from build123d import *

# Parameters (mm, degrees)
SKETCH_1_W      = 50
SKETCH_1_H      = 50
SKETCH_1_R      = 2
SKETCH_1_R_2    = 23.5
EXTRUDE_1_DEPTH = 12
FILLET_1_R      = 5


with BuildPart() as part:
    # 草图1 → 凸台-拉伸1 (new body)
    with BuildSketch(Plane.XY):
        with Locations((-26.20618851, -18.866504484)):
            Rectangle(SKETCH_1_W, SKETCH_1_H)
        with Locations((-46.70618851, -39.366504484)):
            Circle(SKETCH_1_R, mode=Mode.SUBTRACT)
        with Locations((-5.70618851, -39.366504484)):
            Circle(SKETCH_1_R, mode=Mode.SUBTRACT)
        with Locations((-5.70618851, 1.633495516)):
            Circle(SKETCH_1_R, mode=Mode.SUBTRACT)
        with Locations((-46.70618851, 1.633495516)):
            Circle(SKETCH_1_R, mode=Mode.SUBTRACT)
        with Locations((-26.20618851, -18.866504484)):
            Circle(SKETCH_1_R_2, mode=Mode.SUBTRACT)
    extrude(amount=EXTRUDE_1_DEPTH)

    # 圆角1
    fillet_1_edges = [part.edges().sort_by_distance(p)[0] for p in [
        (-51.20618851, 6.133495516, 6),
        (-1.20618851, 6.133495516, 6),
        (-1.20618851, -43.866504484, 6),
        (-51.20618851, -43.866504484, 6),
    ]]
    fillet(fillet_1_edges, radius=FILLET_1_R)


solid = part.part
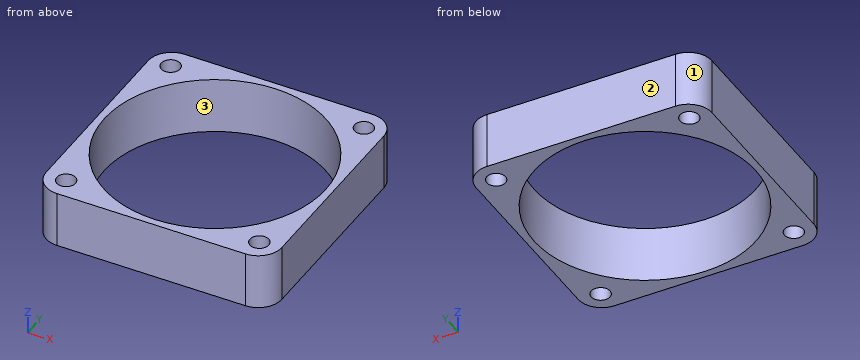
Verification items for the finished model (mm, model axes). Face numbers are marked on the shaded views. Round coordinates to 2 decimals unless told otherwise and drop trailing zeros. Loops run counter-clockwise (first coordinate to the right, second up) from the corner with the lowest first, then second, coordinate; pieces in that order, holes last. Notation, with made-up numbers: (85.25, -10.5) - (109.25, -10.5) arc R13 cw to (109.25, 3.5) - close; hole circle Ø4 at (32.5, -3.5). An arc over 180 degrees is marked (long way). Answer in a Markdown table with one row per item. Add a question column.
Q1. Section check B-B on x = -15. Enter the section's corners in (y, z).
Q2. Section check C-C on z = 2.5. Enter the section's corners in (x, y), plus the area to 3 significant figures.
Q3. Material ranges on line 1 (X direction, y = 2.5, z = 0.5); line 2 (X direction, y = -37, z = 5); line 3 (Y direction, x = -16, z = 3), recorded low to high.
Q4. Gauge pin test, flat end, axial feed: pin 1 (3.5 mm diameter, centred on x = -5.71, y = -39.37, fed in from -Z). Record the tip position at first contact, or that the pin passes through.
Q5. Section check A-A on y = -31. Enter the section's corners in (x, z), plus the area to 3 significant figures.
Q6. Release check for a two-part mould opening along X. For the marked faces 1, 2 and 3 record: pulls with the +X half, pulls with the -X half, needs draft (parallel to the pull), parting line crosses it, or undercut.
Found:
| question | item | result |
|---|---|---|
| 1 | outline | (-43.87, 0) - (-39.52, 0) - (-39.52, 12) - (-43.87, 12) - close; (1.79, 0) - (6.13, 0) - (6.13, 12) - (1.79, 12) - close |
| 2 | outline | (-51.21, -38.87) arc R5 ccw to (-46.21, -43.87) - (-6.21, -43.87) arc R5 ccw to (-1.21, -38.87) - (-1.21, 1.13) arc R5 ccw to (-6.21, 6.13) - (-46.21, 6.13) arc R5 ccw to (-51.21, 1.13) - close; hole circle Ø47 at (-26.21, -18.87); hole circle Ø4 at (-46.71, -39.37); hole circle Ø4 at (-46.71, 1.63); hole circle Ø4 at (-5.71, -39.37); hole circle Ø4 at (-5.71, 1.63) |
| 2 | area | 693 mm² |
| 3 | line 1 | x = -51.02 to -48.51, -44.9 to -35.99, -16.42 to -7.51, -3.9 to -1.4 |
| 3 | line 2 | x = -51.21 to -41.15, -11.26 to -1.21 |
| 3 | line 3 | y = -43.87 to -40.03, 2.3 to 6.13 |
| 4 | pin 1 | passes through |
| 5 | outline | (-51.21, 0) - (-46.33, 0) - (-46.33, 12) - (-51.21, 12) - close; (-6.08, 0) - (-1.21, 0) - (-1.21, 12) - (-6.08, 12) - close |
| 5 | area | 117 mm² |
| 6 | face 1 | pulls with the -X half |
| 6 | face 2 | needs draft |
| 6 | face 3 | undercut |
